```python
from build123d import *

# Parameters (mm, degrees)
BOSS_EXTRUDE1_DEPTH = 10
FILLET1_R           = 5
BOSS_EXTRUDE2_DEPTH = 35
FILLET2_R           = 5


with BuildPart() as part:
    # Sketch1 → Boss-Extrude1 (new body)
    with BuildSketch(Plane(origin=(0, 0, 0), x_dir=(0, 0, -1), z_dir=(1, 0, 0))):
        with BuildLine():
            Line((-45, 0), (-36.39286513, 40))
            ThreePointArc((-36.39286513, 40), (0, 36.128824769), (36.39286513, 40))
            Line((36.39286513, 40), (45, 0))
            Line((45, 0), (34.771110854, 0))
            Line((34.771110854, 0), (28.662747002, 28.387443413))
            ThreePointArc((28.662747002, 28.387443413), (0, 26.128824769), (-28.662747002, 28.387443413))
            Line((-28.662747002, 28.387443413), (-34.771110854, 0))
            Line((-34.771110854, 0), (-45, 0))
        make_face()
    extrude(amount=BOSS_EXTRUDE1_DEPTH)

    # Fillet1
    fillet1_edges = [part.edges().sort_by_distance(p)[0] for p in [
        (5, 40, -36.39286513),
    ]]
    fillet(fillet1_edges, radius=FILLET1_R)


with BuildPart() as body_2:
    # Mirror3: mirrored copy
    add(part.part.mirror(Plane(origin=(45, 0, 0), x_dir=(0, 0, 1), z_dir=(1, 0, 0))))


with BuildPart() as part_1:
    add(part.part)

    add(body_2.part)  # Boss-Extrude2 merges body 2
    # Sketch2 → Boss-Extrude2 (add, symmetric)
    with BuildSketch(Plane(origin=(45, 0, 0), x_dir=(0, 0, -1), z_dir=(1, 0, 0))):
        with BuildLine():
            Line((-48, 23), (48, 23))
            Line((48, 23), (66.416945106, 106))
            Line((66.416945106, 106), (46.416945106, 108.51539025))
            Line((46.416945106, 108.51539025), (45.96709586, 106.741704173))
            Line((45.96709586, 106.741704173), (34.965043573, 63.362311747))
            ThreePointArc((34.965043573, 63.362311747), (25.373507712, 48.690171483), (8.793664269, 43))
            Line((8.793664269, 43), (-43, 43))
            ThreePointArc((-43, 43), (-46.535533906, 41.535533906), (-48, 38))
            Line((-48, 38), (-48, 23))
        make_face()
    extrude(amount=BOSS_EXTRUDE2_DEPTH, both=True)

    # Fillet2
    fillet2_edges = [part_1.edges().sort_by_distance(p)[0] for p in [
        (45, 108.51539025, -46.416945106),
    ]]
    fillet(fillet2_edges, radius=FILLET2_R)


solid = part_1.part
```
Here's how the part is built. I have some questions about the finished solid (model axes, mm). A direction names the side the tool comes from. Give positions to 0.01 mm unless a question says otherwise; leave off trailing zeros. Loops run counter-clockwise (first coordinate to the right, second up) from the corner with the lowest first, then second, coordinate; pieces in that order, holes last. Notation, with made-up numbers: M 12.5,0 L 48.5,0 A21 ccw 48.5,11 Z; hole C 36,44 d10. An arc over 180 degrees is marked long. Use one line per item in the form item = value. Start each with the question number.
Q1. If we section it at B-B (z = -43): Write out the boundary of the cut face in (x, y), then the cut area to 3 significant figures.
Q2. Thinking about a two-plate mould opening in Z: for faces 1 (the flat face through (45.49, 63.92, -57.08)), 2 (the cylindrical face through (85.07, 26.13, -0.4)), 3 (the flat face through (45.49, 84.08, -40.22)), 4 (the flat face through (80, 12, -38)), which applies, +Z half, -Z half, draft (parallel to the pull), parting line (faces both ways), or undercut?
Q3. I need wall thicknesses on line 1 along Y through (x, z) = (57, 18.5); line 2 along X through (y, z) = (10.5, -35); line 3 along X through (y, z) = (42.5, -46). Which ranges of each line are inside material? Lowest first, please.
Q4. Will these pins go through, and if not, where does the flat tip stop? pin 1 Ø1 at (x, z) = (65.5, -18) entering from +Y (3 decimals); pin 2 Ø8 at (x, z) = (44, 28) entering from +Y; pin 3 Ø5 at (x, y) = (80, 65.5) entering from -Z.
Q5. If we section it at D-D (x = 81.5): Write out the boundary of the cut face in (y, z).
Q6. Which directions (+Z, -Z, +X, -X, +Y, -Y) give clear straight access to the entire face, cutting with the end or side of a thin tool? Please do faces 5 (the flat face through (85.07, 14, -31.76)), 6 (the cylindrical face through (4.93, 36.153, 2.909)), 7 (the cylindrical face through (85.07, 36.153, 2.909)), 8 (the flat face through (4.93, 14.392, 31.674)), 9 (the flat face through (10, 12, -38)).
Q7. If we section it at A-A (y = 13): Write out the boundary of the cut face in (x, z).
Q8. If we section it at C-C (z = -24): Write out the boundary of the cut face in (x, y).
Taken from the geometry:
q1.outline = M 0,0 L 10,0 L 10,9.29 L 0,9.29 Z; M 10,23 L 80,23 L 80,95.04 L 10,95.04 Z; M 80,0 L 90,0 L 90,9.29 L 80,9.29 Z
q1.area = 5,230 mm^2
q2.face_1 = -Z half
q2.face_2 = undercut
q2.face_3 = +Z half
q2.face_4 = draft
q3.line_1 = 23 to 43
q3.line_2 = 0 to 10, 80 to 90
q3.line_3 = 10 to 80
q4.pin_1 = 44.805
q4.pin_2 = 43
q4.pin_3 = -57.99
q5.outline = M 0,-45 L 35.18,-37.43 A5 ccw 39.04,-31.63 A173 cw 40,36.39 L 0,45 L 0,34.77 L 28.39,28.66 A183 ccw 28.39,-28.66 L 0,-34.77 Z
q6.face_5 = +X, -Y
q6.face_6 = -X, +Y
q6.face_7 = +X, +Y
q6.face_8 = -X, -Y
q6.face_9 = +Z, -Z, -Y
q7.outline = M 0,-42.2 L 10,-42.2 L 10,-31.97 L 0,-31.97 Z; M 0,31.97 L 10,31.97 L 10,42.2 L 0,42.2 Z; M 80,-42.2 L 90,-42.2 L 90,-31.97 L 80,-31.97 Z; M 80,31.97 L 90,31.97 L 90,42.2 L 80,42.2 Z
q8.outline = M 0,27.71 L 10,27.71 L 10,23 L 80,23 L 80,27.71 L 90,27.71 L 90,37.8 L 80,37.8 L 80,47.69 L 10,47.69 L 10,37.8 L 0,37.8 Z
